Input: part model. Units: mm. Frame: model coordinates. Face numbers are marked on the shaded views. A direction names the side the tool comes from. Give positions to 0.01 mm unless a question says otherwise; leave off trailing zeros. Loops run counter-clockwise (first coordinate to the right, second up) from the corner with the lowest first, then second, coordinate; pieces in that order, holes last.
from build123d import *

# Parameters (mm, degrees)
SKETCH1_W            = 30
SKETCH1_H            = 15
BOSS_EXTRUDE1_DEPTH  = 45
SKETCH2_W            = 6
SKETCH2_H            = 15
BOSS_EXTRUDE2_DEPTH  = 7.5
BOSS_EXTRUDE3_DEPTH  = 6
BOSS_EXTRUDE4_START  = -24
BOSS_EXTRUDE4_DEPTH  = 6
SKETCH4_R            = 3
CUT_EXTRUDE1_DEPTH   = 30
SKETCH18_W           = 30
SKETCH18_H           = 15
BOSS_EXTRUDE10_DEPTH = 20
BOSS_EXTRUDE11_DEPTH = 30
SKETCH19_W           = 5
SKETCH19_H           = 15
BOSS_EXTRUDE12_DEPTH = 7.5
CUT_EXTRUDE7_REACH   = 88.894
SKETCH22_W           = 4
SKETCH22_H           = 25
SKETCH23_R           = 3
CUT_EXTRUDE8_DEPTH   = 83.00662079
BOSS_EXTRUDE15_DEPTH = 5
BOSS_EXTRUDE16_START = -15
BOSS_EXTRUDE16_DEPTH = 5
SKETCH25_R           = 3
CUT_EXTRUDE10_DEPTH  = 20


with BuildPart() as part:
    # Sketch1 → Boss-Extrude1 (new body)
    with BuildSketch(Plane.XY):
        with Locations((15, 7.5)):
            Rectangle(SKETCH1_W, SKETCH1_H)
    extrude(amount=BOSS_EXTRUDE1_DEPTH)

    # Sketch2 → Boss-Extrude2 (add)
    with BuildSketch(Plane(origin=(0, 0, 0), x_dir=(-1, 0, 0), z_dir=(0, 0, -1))):
        with Locations((-27, 7.5)):
            Rectangle(SKETCH2_W, SKETCH2_H)
        with Locations((-3, 7.5)):
            Rectangle(SKETCH2_W, SKETCH2_H)
    extrude(amount=BOSS_EXTRUDE2_DEPTH)

    # Sketch3 → Boss-Extrude3 (add)
    with BuildSketch(Plane(origin=(30, 0, 0), x_dir=(0, 0, -1), z_dir=(1, 0, 0))):
        with BuildLine():
            Line((7.5, 15), (7.5, 0))
            ThreePointArc((7.5, 0), (15, 7.5), (7.5, 15))
        make_face()
    extrude(amount=-BOSS_EXTRUDE3_DEPTH)

    # Sketch3<2> → Boss-Extrude4 (add)
    with BuildSketch(Plane(origin=(30, 0, 0), x_dir=(0, 0, -1), z_dir=(1, 0, 0)).offset(BOSS_EXTRUDE4_START)):
        with BuildLine():
            Line((7.5, 15), (7.5, 0))
            ThreePointArc((7.5, 0), (15, 7.5), (7.5, 15))
        make_face()
    extrude(amount=-BOSS_EXTRUDE4_DEPTH)

    # Sketch4 → Cut-Extrude1 (cut)
    with BuildSketch(Plane.ZY):
        with Locations((-7.5, 7.5)):
            Circle(SKETCH4_R)
    extrude(amount=-CUT_EXTRUDE1_DEPTH, mode=Mode.SUBTRACT)



with BuildPart() as body_2:
    # Sketch18 → Boss-Extrude10 (new body)
    with BuildSketch(Plane(origin=(0, -19.485571585, 33.75), x_dir=(1, 0, 0), z_dir=(0, -0.500000000000001, 0.866025403784438))):
        with Locations((15, 30)):
            Rectangle(SKETCH18_W, SKETCH18_H)
    extrude(amount=BOSS_EXTRUDE10_DEPTH)


with BuildPart() as part_1:
    add(part.part)

    add(body_2.part)  # Boss-Extrude11 merges body 2
    # 3DSketch1 → Boss-Extrude11 (add)
    with BuildSketch(Plane(origin=(30, 0, 45), x_dir=(0, 1, 0), z_dir=(1, 0, 0))):
        Polygon((0, 0), (15, 0), (12.990381057, 7.5), align=None)
    extrude(amount=-BOSS_EXTRUDE11_DEPTH)

    # Sketch19 → Boss-Extrude12 (add)
    with BuildSketch(Plane(origin=(0, -29.485571585, 51.070508076), x_dir=(1, 0, 0), z_dir=(0, -0.5000000000000009, 0.8660254037844383))):
        with Locations((7.5, 30)):
            Rectangle(SKETCH19_W, SKETCH19_H)
        with Locations((22.5, 30)):
            Rectangle(SKETCH19_W, SKETCH19_H)
    extrude(amount=BOSS_EXTRUDE12_DEPTH)

    # Sketch22 → Cut-Extrude7 (cut, up to next)
    with BuildSketch(Plane(origin=(0, 15, 0), x_dir=(1, 0, 0), z_dir=(0, 1, 0)), mode=Mode.PRIVATE) as cut_extrude7_sk1:
        with Locations((2, -32.5)):
            Rectangle(SKETCH22_W, SKETCH22_H)
    cut_extrude7_tool1 = extrude(cut_extrude7_sk1.sketch, amount=-CUT_EXTRUDE7_REACH, mode=Mode.PRIVATE) & part_1.part
    # Sketch22 → Cut-Extrude7 (cut, up to next)
    with BuildSketch(Plane(origin=(0, 15, 0), x_dir=(1, 0, 0), z_dir=(0, 1, 0)), mode=Mode.PRIVATE) as cut_extrude7_sk2:
        with Locations((28, -32.5)):
            Rectangle(SKETCH22_W, SKETCH22_H)
    cut_extrude7_tool2 = extrude(cut_extrude7_sk2.sketch, amount=-CUT_EXTRUDE7_REACH, mode=Mode.PRIVATE) & part_1.part
    add(cut_extrude7_tool1.solids().sort_by_distance((2, 15, 32.5))[0], mode=Mode.SUBTRACT)
    add(cut_extrude7_tool2.solids().sort_by_distance((28, 15, 32.5))[0], mode=Mode.SUBTRACT)

    # Sketch23 → Cut-Extrude8 (cut, through all)
    with BuildSketch(Plane.ZY.offset(-4)):
        with Locations((32.5, 7.5)):
            Circle(SKETCH23_R)
    extrude(amount=-CUT_EXTRUDE8_DEPTH, mode=Mode.SUBTRACT)

    # Sketch24 → Boss-Extrude15 (add)
    with BuildSketch(Plane(origin=(25, 0, 0), x_dir=(0, 0, -1), z_dir=(1, 0, 0))):
        with BuildLine():
            Line((-76.315698604, -0.759618943), (-68.815698604, -13.75))
            ThreePointArc((-68.815698604, -13.75), (-79.060889132, -11.004809472), (-76.315698604, -0.759618943))
        make_face()
    extrude(amount=-BOSS_EXTRUDE15_DEPTH)

    # Sketch24<2> → Boss-Extrude16 (add)
    with BuildSketch(Plane(origin=(25, 0, 0), x_dir=(0, 0, -1), z_dir=(1, 0, 0)).offset(BOSS_EXTRUDE16_START)):
        with BuildLine():
            Line((-76.315698604, -0.759618943), (-68.815698604, -13.75))
            ThreePointArc((-68.815698604, -13.75), (-79.060889132, -11.004809472), (-76.315698604, -0.759618943))
        make_face()
    extrude(amount=-BOSS_EXTRUDE16_DEPTH)

    # Sketch25 → Cut-Extrude10 (cut)
    with BuildSketch(Plane(origin=(25, 0, 0), x_dir=(0, 0, -1), z_dir=(1, 0, 0))):
        with Locations((-72.565698604, -7.254809472)):
            Circle(SKETCH25_R)
    extrude(amount=-CUT_EXTRUDE10_DEPTH, mode=Mode.SUBTRACT)


solid = part_1.part
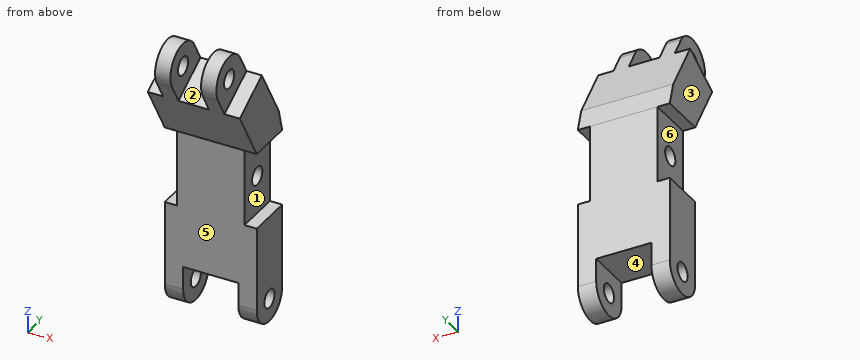
(1) Cut plane C-C (y = 7.5). Return the cut outline in (x, z).
Values follow:
outline: (0, -15) - (6, -15) - (6, -10.5) - (0, -10.5) - close; (0, -4.5) - (6, -4.5) - (6, 0) - (24, 0) - (24, -4.5) - (30, -4.5) - (30, 20) - (26, 20) - (26, 29.5) - (4, 29.5) - (4, 20) - (0, 20) - close; (0, 45) - (4, 45) - (4, 35.5) - (26, 35.5) - (26, 45) - (30, 45) - (30, 62.01) - (0, 62.01) - close; (24, -15) - (30, -15) - (30, -10.5) - (24, -10.5) - close
(2) Cut plane D-D (x = 9). Return the cut outline in (y, z).
Values follow:
outline: (-13.75, 68.82) - (0, 45) - (0, 0) - (15, 0) - (15, 45) - (12.99, 52.5) - (-0.76, 76.32) arc R7.5 ccw to start; hole circle Ø6 at (-7.25, 72.57); hole circle Ø6 at (7.5, 32.5)
(3) Reachability of the marked faces 1, 2 and 3 from +Z, -Z, +X, -X, +Y, -Y: full face, straight path, thin tool, end or side. Return the list, or none.
Values follow:
face 1: +X, +Y, -Y
face 2: +Z, -Y
face 3: +Z, -Z, -X, +Y, -Y
(4) Cut plane B-B (x = 16). Return the cut outline in (y, z), and give its area (3 significant figures).
Values follow:
outline: (-10, 62.32) - (0, 45) - (0, 0) - (15, 0) - (15, 45) - (12.99, 52.5) - (2.99, 69.82) - close; hole circle Ø6 at (7.5, 32.5)
area: 1,000 mm2
(5) Ray query, probe 1 along X at (y, z) = (-5.5, 69); probe 2 along Z at (x, y) = (28, 9.25); probe 3 along Y at (x, z) = (17.25, 32.5). Return the intervals inside material, ascending.
Values follow:
probe 1: x = 5 to 10, 20 to 25
probe 2: z = -14.79 to -9.94, -5.06 to 20, 45 to 58.98
probe 3: y = 0 to 4.5, 10.5 to 15
(6) Mould query, pull axis Z, two halves, no side actions, for the marked faces 4, 5 and 6. Classes: +Z half, -Z half, draft (parallel to the pull), parting line (faces both ways), or undercut.
Values follow:
face 4: -Z half
face 5: draft
face 6: undercut
(7) Cut plane A-A (z = 32.5). Return the cut outline in (x, y).
Values follow:
outline: (4, 0) - (26, 0) - (26, 4.5) - (4, 4.5) - close; (4, 10.5) - (26, 10.5) - (26, 15) - (4, 15) - close
(8) Pin query (flat end, axial travel): pin 1 Ø5 at (x, z) = (21.5, 6) entering from -Y; pin 2 Ø12 at (x, y) = (19, 8) entering from +Z; pin 3 Ø9 at (y, z) = (-10, 75) entering from +X. Return the tip coordinate at first contact, or that it passes through.
Values follow:
pin 1: stops at y = 0
pin 2: stops at z = 71.39
pin 3: stops at x = 25
